from build123d import *

# Parameters (mm, degrees)
SKETCH1_W           = 37.084
SKETCH1_H           = 9.144
BOSS_EXTRUDE1_DEPTH = 4.318
SKETCH2_W           = 34.544
SKETCH2_H           = 6.604
CUT_EXTRUDE3_DEPTH  = 2.667
FILLET1_R           = 1.27
FILLET2_R           = 1.016
SKETCH11_R          = 0.889
CUT_EXTRUDE4_DEPTH  = 20.282682308


with BuildPart() as part:
    # Sketch1 → Boss-Extrude1 (new body)
    with BuildSketch(Plane(origin=(0, 0, 0), x_dir=(1, 0, 0), z_dir=(0, 1, 0))):
        Rectangle(SKETCH1_W, SKETCH1_H)
    extrude(amount=BOSS_EXTRUDE1_DEPTH)

    # Sketch2 → Cut-Extrude3 (cut)
    with BuildSketch(Plane(origin=(0, 4.318, 0), x_dir=(1, 0, 0), z_dir=(0, 1, 0))):
        Rectangle(SKETCH2_W, SKETCH2_H)
    extrude(amount=-CUT_EXTRUDE3_DEPTH, mode=Mode.SUBTRACT)

    # Fillet1
    fillet1_edges = [part.edges().sort_by_distance(p)[0] for p in [
        (0, 0, 4.572),
        (-18.542, 0, 0),
        (0, 0, -4.572),
        (18.542, 0, 0),
        (18.542, 2.159, 4.572),
        (-18.542, 2.159, 4.572),
        (-18.542, 2.159, -4.572),
        (18.542, 2.159, -4.572),
    ]]
    fillet(fillet1_edges, radius=FILLET1_R)

    # Fillet2
    fillet2_edges = [part.edges().sort_by_distance(p)[0] for p in [
        (-17.272, 2.9845, -3.302),
        (-17.272, 2.9845, 3.302),
        (17.272, 2.9845, 3.302),
        (17.272, 2.9845, -3.302),
    ]]
    fillet(fillet2_edges, radius=FILLET2_R)

    # Sketch11 → Cut-Extrude4 (cut, through all)
    with BuildSketch(Plane(origin=(0, 1.651, 0), x_dir=(1, 0, 0), z_dir=(0, 1, 0))):
        with Locations(Location((-16.002, 0, 0), (0, 0, 270))):
            Circle(SKETCH11_R)
        with Locations(Location((16.002, 0, 0), (0, 0, 270))):
            Circle(SKETCH11_R)
    extrude(amount=-CUT_EXTRUDE4_DEPTH, mode=Mode.SUBTRACT)


solid = part.part
The model under review builds one solid part; all positions refer to its coordinate system, in mm. A direction names the side the tool comes from. Round coordinates to 2 decimals unless told otherwise and drop trailing zeros. Write each loop counter-clockwise with the first axis right and the second up, starting at its lowest first coordinate (ties: lowest second). Pieces come first, ordered by that corner, then holes. Notation, with made-up numbers: M 21.5,-27.75 L 50.5,-27.75 A17 cw 50.5,-7.75 Z; hole C 75.5,-27.75 d4. An arc over 180 degrees is marked long. Use a Markdown table: item, result. Add a question column.
Q1. Insertion check: pin 1 (3.5 mm diameter, centred on x = -5.5, z = 1.5, fed in from +Y). The pin has a flat end and moves straight along its axis. Give the tip position at first contact, or say it passes through.
Q2. To check wall thickness, follow line 1 (Z direction, x = -15.5, y = 3.55); line 2 (X direction, y = 0.45, z = 0); line 3 (X direction, y = 1.4, z = 0.75). State the ranges of each line that lie inside material, in increasing order.
Q3. We need section B-B, the plane y = 4. State the section outline as (x, z) points.
Q4. Machinability: for faces 4 (the face through (-16.97, 2.97, 3.01)), 5 (the face through (0, 0, 0)), which of the approach directions +Z, -Z, +X, -X, +Y, -Y give a long, thin tool a straight path to every point of the face, cutting with its end or side? Answer none if there is none.
Q5. We need section D-D, the plane x = -12.5. State the section outline as (y, z) points.
Q6. The part is to be moulded in two halves that separate along X. For faces 1 (the face through (0, 3, 3.302)), 2 (the face through (-18.18, 2.82, 4.19)), 3 (the face through (0, 4.318, -4)), say which applies: pulls with the +X half, pulls with the -X half, needs draft (parallel to the pull), parting line crosses it, or undercut.
Q7. We need section A-A, the plane z = 0. State the section outline as (x, y) points.
Q8. We need section C-C, the plane z = 1.5. State the section outline as (x, y) points, plus the area to 3 significant figures.
Findings below:
| question | item | result |
|---|---|---|
| 1 | pin 1 | stops at y = 1.65 |
| 2 | line 1 | z = -4.57 to -3.3, 3.3 to 4.57 |
| 2 | line 2 | x = -18.24 to -16.89, -15.11 to 15.11, 16.89 to 18.24 |
| 2 | line 3 | x = -18.54 to -16.48, -15.52 to 15.52, 16.48 to 18.54 |
| 3 | outline | M -18.54,-3.3 A1.27 ccw -17.27,-4.57 L 17.27,-4.57 A1.27 ccw 18.54,-3.3 L 18.54,3.3 A1.27 ccw 17.27,4.57 L -17.27,4.57 A1.27 ccw -18.54,3.3 Z; hole M -17.27,-2.29 A1.02 ccw -16.26,-3.3 L 16.26,-3.3 A1.02 ccw 17.27,-2.29 L 17.27,2.29 A1.02 ccw 16.26,3.3 L -16.26,3.3 A1.02 ccw -17.27,2.29 Z |
| 4 | face 4 | +Y |
| 4 | face 5 | +Z, -Z, +X, -X, -Y |
| 5 | outline | M 0,-3.3 A1.27 ccw 1.27,-4.57 L 4.32,-4.57 L 4.32,-3.3 L 1.65,-3.3 L 1.65,3.3 L 4.32,3.3 L 4.32,4.57 L 1.27,4.57 A1.27 ccw 0,3.3 Z |
| 6 | face 1 | undercut |
| 6 | face 2 | pulls with the -X half |
| 6 | face 3 | needs draft |
| 7 | outline | M -18.54,1.27 A1.27 ccw -17.27,0 L -16.89,0 L -16.89,1.65 L -17.27,1.65 L -17.27,4.32 L -18.54,4.32 Z; M -15.11,0 L 15.11,0 L 15.11,1.65 L -15.11,1.65 Z; M 16.89,0 L 17.27,0 A1.27 ccw 18.54,1.27 L 18.54,4.32 L 17.27,4.32 L 17.27,1.65 L 16.89,1.65 Z |
| 8 | outline | M -18.54,1.27 A1.27 ccw -17.27,0 L 17.27,0 A1.27 ccw 18.54,1.27 L 18.54,4.32 L 17.27,4.32 L 17.27,1.65 L -17.27,1.65 L -17.27,4.32 L -18.54,4.32 Z |
| 8 | area | 67.3 mm² |
